Input: dimensioned drawing with shaded views. Units: mm. Origin: part minimum x, y, z. A direction names the side the tool comes from. Round coordinates to 2 decimals unless told otherwise and drop trailing zeros. Order: outer loops, then holes, each group sorted by start corner. A loop starts at its lowest first (then second) coordinate and runs counter-clockwise, first axis right, second up. Notation, with made-up numbers: M 25,52 L 45,52 A24 ccw 45,68 Z; hole C 13.5,-33.75 d6. An arc over 180 degrees is marked long. Answer as CSV lines item,"result". Start each with the question number.
Item 1: Section query B-B on z = 9. Return the cut outline in (x, y), plus the area to 3 significant figures.
Item 2: Pull-direction query (X, two-part tool) for the marked faces 1, 2 and 3; classes: +X half, -X half, draft (parallel to the pull), parting line (faces both ways), or undercut.
Item 3: Section query D-D on z = 1.5. Return the cut outline in (x, y), plus the area to 3 significant figures.
Item 4: First-contact query: P1, Ø2.5, axis at x = 34.5, y = 4.5, coming from the +Z side. Flat tip, straight axial feed; report the tip coordinate or a pass-through.
Item 5: Set-up query: the marked faces 4 and 5. Return all of +Z, -Z, +X, -X, +Y, -Y with unobstructed straight access to the full face (end or side cutting, diameter ignored); none if empty.
Item 6: Section query C-C on y = 4. Return the cut outline in (x, z), plus the area to 3 significant figures.
Item 7: Line query: line 1 (Y direction, x = 52, z = 4.25); line 2 (X direction, y = 2.5, z = 8.5); line 3 (X direction, y = 3.25, z = 1.5). Output: solid intervals per line, ascending. Write a range as [from, to].
Item 8: Section query A-A on x = 52. Return the cut outline in (y, z).
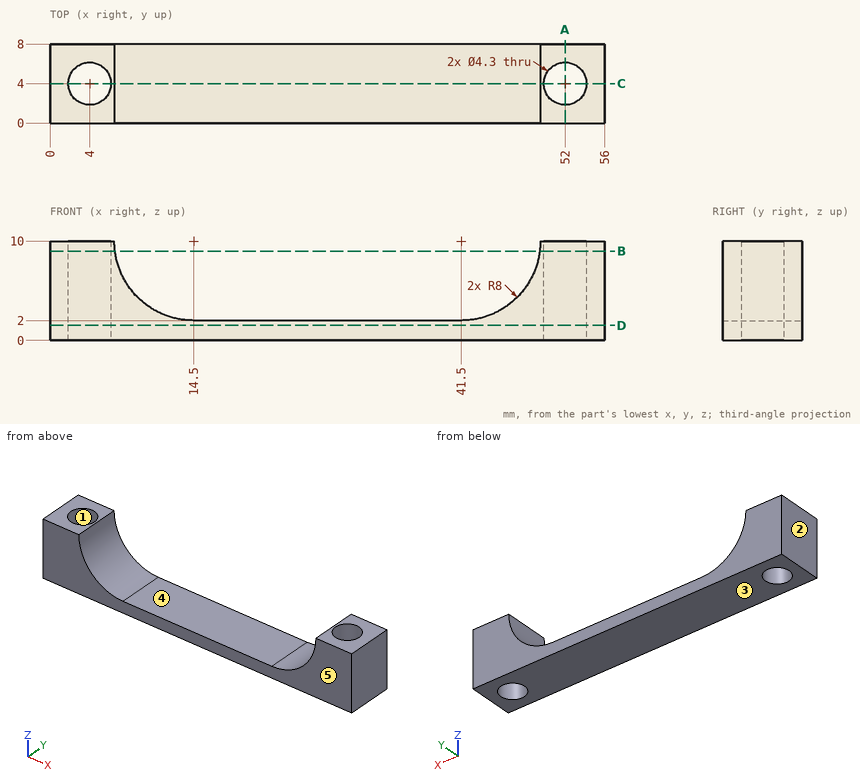
Results:
1,outline,"M 0,0 L 6.56,0 L 6.56,8 L 0,8 Z; M 49.44,0 L 56,0 L 56,8 L 49.44,8 Z; hole C 4,4 d4.3; hole C 52,4 d4.3"
1,area,"76.0 mm^2"
2,face 1,"undercut"
2,face 2,"-X half"
2,face 3,"draft"
3,outline,"M 0,0 L 56,0 L 56,8 L 0,8 Z; hole C 4,4 d4.3; hole C 52,4 d4.3"
3,area,"419 mm^2"
4,P1,"z = 2"
5,face 4,"+Z, +Y, -Y"
5,face 5,"+Z, -Z, +X, -X, -Y"
6,outline,"M 0,0 L 1.85,0 L 1.85,10 L 0,10 Z; M 6.15,0 L 49.85,0 L 49.85,10 L 49.5,10 A8 cw 41.5,2 L 14.5,2 A8 cw 6.5,10 L 6.15,10 Z; M 54.15,0 L 56,0 L 56,10 L 54.15,10 Z"
6,area,"157 mm^2"
7,line 1,"[0, 1.85], [6.15, 8]"
7,line 2,"[0, 2.46], [5.54, 6.64], [49.36, 50.46], [53.54, 56]"
7,line 3,"[0, 1.99], [6.01, 49.99], [54.01, 56]"
8,outline,"M 0,0 L 1.85,0 L 1.85,10 L 0,10 Z; M 6.15,0 L 8,0 L 8,10 L 6.15,10 Z"
